Input: part model. Units: mm. Frame: model coordinates. A direction names the side the tool comes from. Coordinates: 2 decimals unless noted, no trailing zeros. Loops run counter-clockwise (first coordinate to the right, second up) from the corner with the lowest first, then second, coordinate; pieces in that order, holes last. Notation, with made-up numbers: (78.25, 77) - (130.25, 77) arc R20 cw to (130.25, 101) - close; hole circle Ø3 at (11.25, 42). An arc over 180 degrees is marked (long way). Use a Markdown table: item, result. Add a question column.
1. Ray query, L1, parallel to X at y = 30.5, z = 28.5; L2, parallel to X at y = 30, z = 27; L3, parallel to Z at x = -11.5, y = 20. Return the intervals inside material, ascending. Write a range as [from, to].
2. Section query C-C on x = -62. Return the cut outline in (y, z).
3. Access query for faces 1 (the face through (-6.595, 22.941, 28.656)), 2 (the face through (-76.2, 19, 13)). Directions: +Z, -Z, +X, -X, +Y, -Y. A direction counts if a zero-diameter tool reaches every point of the face in a straight line with its end or side. Return the directions, or none.
4. Section query D-D on x = -44.5. Return the cut outline in (y, z).
5. Contact query for flat-ended pins moving along their axis: P1, Ø6, axis at y = 25.5, z = 19.5, coming from the +X side; P2, Ø1.5, axis at x = -55.5, y = 12.5, coming from the +Z side. Output: stop coordinate, or through.
6. Section query A-A on z = 28. Return the cut outline in (x, y) (3 decimals), then the cut area to 3 significant figures.
7. Section query B-B on y = 27. Return the cut outline in (x, z), then the cut area to 3 significant figures.
8. Draft query along Y for faces 3 (the face through (-39, 38.1, 13)), 4 (the face through (-48, 29, 32.004)), 5 (the face through (-22.71, 7.09, 28.66)). Return one class per face: released by +Y, released by -Y, zero draft, split by the parting line, or undercut.
```python
from build123d import *

# Parameters (mm, degrees)
F0_W     = 76.2
F0_H     = 38.1
F1_DEPTH = 25.4
F2_R     = 6.35
F3_DEPTH = 6.604


with BuildPart() as f1:
    # F0 (on Top) → F1 (new body)
    with BuildSketch(Plane.XY):
        with Locations((-38.1, 19.05)):
            Rectangle(F0_W, F0_H)
    extrude(amount=F1_DEPTH)

    # F2 (on face) → F3 (join)
    with BuildSketch(Plane.XY.offset(25.4)):
        with Locations((-66.675, 28.575)):
            Circle(F2_R)
        with Locations((-47.625, 28.575)):
            Circle(F2_R)
        with Locations((-28.575, 28.575)):
            Circle(F2_R)
        with Locations((-9.525, 28.575)):
            Circle(F2_R)
        with Locations((-9.525, 9.525)):
            Circle(F2_R)
        with Locations((-28.575, 9.525)):
            Circle(F2_R)
        with Locations((-47.625, 9.525)):
            Circle(F2_R)
        with Locations((-66.675, 9.525)):
            Circle(F2_R)
    extrude(amount=F3_DEPTH)


solid = f1.part
```
Resolved:
| question | item | result |
|---|---|---|
| 1 | L1 | [-72.73, -60.62], [-53.68, -41.57], [-34.63, -22.52], [-15.58, -3.47] |
| 1 | L2 | [-72.86, -60.49], [-53.81, -41.44], [-34.76, -22.39], [-15.71, -3.34] |
| 1 | L3 | [0, 25.4] |
| 2 | outline | (0, 0) - (38.1, 0) - (38.1, 25.4) - (32.87, 25.4) - (32.87, 32) - (24.28, 32) - (24.28, 25.4) - (13.82, 25.4) - (13.82, 32) - (5.23, 32) - (5.23, 25.4) - (0, 25.4) - close |
| 3 | face 1 | +Z |
| 3 | face 2 | +Z, -Z, -X, +Y, -Y |
| 4 | outline | (0, 0) - (38.1, 0) - (38.1, 25.4) - (34.1, 25.4) - (34.1, 32) - (23.05, 32) - (23.05, 25.4) - (15.05, 25.4) - (15.05, 32) - (4, 32) - (4, 25.4) - (0, 25.4) - close |
| 5 | P1 | x = 0 |
| 5 | P2 | z = 25.4 |
| 6 | outline | circle Ø12.7 at (-66.675, 9.525); circle Ø12.7 at (-66.675, 28.575); circle Ø12.7 at (-47.625, 9.525); circle Ø12.7 at (-47.625, 28.575); circle Ø12.7 at (-28.575, 9.525); circle Ø12.7 at (-28.575, 28.575); circle Ø12.7 at (-9.525, 9.525); circle Ø12.7 at (-9.525, 28.575) |
| 6 | area | 1,010 mm² |
| 7 | outline | (-76.2, 0) - (0, 0) - (0, 25.4) - (-3.37, 25.4) - (-3.37, 32) - (-15.68, 32) - (-15.68, 25.4) - (-22.42, 25.4) - (-22.42, 32) - (-34.73, 32) - (-34.73, 25.4) - (-41.47, 25.4) - (-41.47, 32) - (-53.78, 32) - (-53.78, 25.4) - (-60.52, 25.4) - (-60.52, 32) - (-72.83, 32) - (-72.83, 25.4) - (-76.2, 25.4) - close |
| 7 | area | 2,260 mm² |
| 8 | face 3 | released by +Y |
| 8 | face 4 | zero draft |
| 8 | face 5 | undercut |
